Read the model definition and answer for the solid it produces. Units are mm, in the model's axes. A direction names the side the tool comes from. Round coordinates to 2 decimals unless told otherwise and drop trailing zeros. Loops run counter-clockwise (first coordinate to the right, second up) from the corner with the lowest first, then second, coordinate; pieces in that order, holes last. Notation, with made-up numbers: M -14.5,80 L 33.5,80 A20 cw 33.5,109 Z; hole C 2.25,8 d2. An arc over 180 degrees is marked long. Write each question's results on one line, items separated by ' | '.
from build123d import *

# Parameters (mm, degrees)
BOSS_EXTRUDE1_DEPTH          = 50.8
CUT_EXTRUDE1_START           = -50.8
CUT_EXTRUDE1_DEPTH           = 34.036
SKETCH10_W                   = 50.546
SKETCH10_H                   = 34.036
CUT_EXTRUDE3_DEPTH           = 20.734311378
CUT_EXTRUDE4_DEPTH           = 2.54
CUT_EXTRUDE5_DEPTH           = 7.874
FILLET1_R                    = 2.54
FILLET2_R                    = 2.54
CUT_EXTRUDE6_DEPTH           = 51.8
F_10_0_1935_DIAMETER_HOLE1_D = 4.9149
FILLET3_R                    = 2.54
CUT_EXTRUDE7_DEPTH           = 5.334
SKETCH18_W                   = 7.62
SKETCH18_H                   = 2.54


with BuildPart() as part:
    # Sketch1 → Boss-Extrude1 (new body)
    with BuildSketch(Plane(origin=(0, 0, 0), x_dir=(1, 0, 0), z_dir=(0, 1, 0))):
        with BuildLine():
            Line((63.017839503, -66.782093), (53.468205472, -26.506342671))
            Line((53.468205472, -26.506342671), (-35.875703335, -47.690346072))
            Line((-35.875703335, -47.690346072), (-26.326069304, -87.966096401))
            ThreePointArc((-26.326069304, -87.966096401), (21.184003401, -89.343908807), (63.017839503, -66.782093))
        make_face()
    extrude(amount=BOSS_EXTRUDE1_DEPTH)

    # Sketch2 → Cut-Extrude1 (cut)
    with BuildSketch(Plane(origin=(0, 50.8, 0), x_dir=(1, 0, 0), z_dir=(0, 1, 0)).offset(CUT_EXTRUDE1_START)):
        Polygon((19.413866358, -81.878324539), (49.046880649, -74.852150244), (42.542248899, -47.418750859), (-6.6401518, -59.08020778), (-0.13552005, -86.513607165), align=None)
    extrude(amount=CUT_EXTRUDE1_DEPTH, mode=Mode.SUBTRACT)

    # Sketch10 → Cut-Extrude3 (cut, through all)
    with BuildSketch(Plane(origin=(19.413866358, 0, 81.878324539), x_dir=(-0.973022607, 0, 0.230709788), z_dir=(-0.230709788, 0, -0.973022607))):
        with Locations((-5.1816, 17.018)):
            Rectangle(SKETCH10_W, SKETCH10_H)
    extrude(amount=-CUT_EXTRUDE3_DEPTH, mode=Mode.SUBTRACT)

    # Sketch11 → Cut-Extrude4 (cut)
    with BuildSketch(Plane.XZ.offset(-34.036)):
        Polygon((4.126655542, 64.024522649), (32.455610184, 56.972208264), (36.418920031, 72.892715879), (8.089965389, 79.945030264), align=None)
    extrude(amount=-CUT_EXTRUDE4_DEPTH, mode=Mode.SUBTRACT)

    # Sketch12 → Cut-Extrude5 (cut)
    with BuildSketch(Plane(origin=(0, 50.8, 0), x_dir=(1, 0, 0), z_dir=(0, 1, 0))):
        Polygon((-3.21042467, -90.775014105), (35.097475372, -81.69196977), (27.186436757, -48.327024572), (-11.121463285, -57.410068908), align=None)
    extrude(amount=-CUT_EXTRUDE5_DEPTH, mode=Mode.SUBTRACT)

    # Fillet1
    fillet1_edges = [part.edges().sort_by_distance(p)[0] for p in [
        (53.468205472, 25.4, 26.506342671),
    ]]
    fillet(fillet1_edges, radius=FILLET1_R)

    # Fillet2
    fillet2_edges = [part.edges().sort_by_distance(p)[0] for p in [
        (-35.875703335, 25.4, 47.690346072),
    ]]
    fillet(fillet2_edges, radius=FILLET2_R)

    # Sketch13 → Cut-Extrude6 (cut, through all)
    with BuildSketch(Plane(origin=(0, 50.8, 0), x_dir=(1, 0, 0), z_dir=(0, 1, 0))):
        Polygon((56.792853338, -82.364213599), (69.150240448, -79.434199297), (54.970742259, -19.631915037), (-50.56134592, -44.654237709), (-47.281500933, -58.487041918), (45.893200136, -36.394733549), align=None)
    extrude(amount=-CUT_EXTRUDE6_DEPTH, mode=Mode.SUBTRACT)

    # #10 (0.1935) Diameter Hole1 (through all)
    with Locations(Plane(origin=(0, 50.8, 0), x_dir=(1, 0, 0), z_dir=(0, 1, 0))):
        with Locations((-9.336173019, -54.694807642), (34.992334459, -45.467652744)):
            Hole(F_10_0_1935_DIAMETER_HOLE1_D / 2)

    # Fillet3
    fillet3_edges = [part.edges().sort_by_distance(p)[0] for p in [
        (-34.059094468, 25.4, 55.35192608),
        (45.893200136, 25.4, 36.394733549),
    ]]
    fillet(fillet3_edges, radius=FILLET3_R)

    # Sketch17 → Cut-Extrude7 (cut)
    with BuildSketch(Plane(origin=(0, 50.8, 0), x_dir=(1, 0, 0), z_dir=(0, 1, 0))):
        Polygon((-5.287837916, -82.013487021), (33.020062126, -72.930442686), (37.24926209, -90.767168294), (-1.058637951, -99.850212629), align=None)
    extrude(amount=-CUT_EXTRUDE7_DEPTH, mode=Mode.SUBTRACT)

    # Sketch18 → Cut-Revolve1 (revolve, cut)
    with BuildSketch(Plane(origin=(0, 0, 0), x_dir=(0, 1, 0), z_dir=(0.999925437, 0, -0.012211508))):
        with Locations((36.576, 90.551)):
            Rectangle(SKETCH18_W, SKETCH18_H)
    revolve(axis=Axis((0, 50.8, 0), (0, -1, 0)), mode=Mode.SUBTRACT)


solid = part.part
Item 1: The mould has two halves that part along X. Classify faces 1 (the face through (10, 50.8, 52)), 2 (the face through (50.553, 25.756, 56.048)), 3 (the face through (-9.016, 25.044, 52.258)): pulls with the +X half, pulls with the -X half, needs draft (parallel to the pull), parting line crosses it, or undercut.
Outcome:
face 1: needs draft | face 2: pulls with the +X half | face 3: undercut
Item 2: Straight lines are drawn through the part: line 1 (Y direction, x = -1, z = 64); line 2 (Y direction, x = 25.5, z = 73); line 3 (Z direction, x = 37, y = 48). For each, find the intervals that lie inside material, in ascending order.
Outcome:
line 1: y = 34.04 to 42.93 | line 2: y = 36.58 to 42.93 | line 3: z = 38.5 to 44.05, 46.88 to 84.04
Item 3: Flat-ended cylindrical pins translate along their axes: pin 1 (4 mm diameter, centred on y = 18, z = 74.5, fed in from -X); pin 2 (5 mm diameter, centred on x = 9.5, z = 88, fed in from +Y); pin 3 (1 mm diameter, centred on y = 43, z = 80.5, fed in from -X). Find the tip coordinate at first contact, or state that the pin passes through.
Outcome:
pin 1: stops at x = -29.99 | pin 2: stops at y = 45.47 | pin 3: stops at x = -28.21
Item 4: The part is cut by section C-C (z = 78.5). Determine the outline of the cut face in (x, y), plus the area to 3 significant figures.
Outcome:
outline: M -28.57,0 L -2.04,0 L -2.04,34.04 L 7.73,34.04 L 7.73,36.58 L 13.89,36.58 L 13.89,34.04 L 42.53,34.04 L 42.53,40.39 L 47.63,40.39 L 47.63,50.8 L 34.34,50.8 L 34.34,42.93 L -6.12,42.93 L -6.12,50.8 L -28.57,50.8 Z | area: 1,810 mm2
Item 5: The part is cut by section B-B (x = -15). Determine the outline of the cut face in (y, z), plus the area to 3 significant figures.
Outcome:
outline: M 0,50.83 L 50.8,50.83 L 50.8,90.59 L 40.39,90.59 L 40.39,88.01 L 32.77,88.01 L 32.77,90.59 L 0,90.59 Z | area: 2,000 mm2
Item 6: For faces 4 (the face through (15.86, 36.63, 87.86)), 5 (the face through (12, 42.926, 69)), 6 (the face through (52, 32.766, 74)), determine the directions among +Z, -Z, +X, -X, +Y, -Y from which every point of the face is accessible in a straight line to the end or side of a thin tool.
Outcome:
face 4: +Z | face 5: +Y | face 6: +Z, +X
Item 7: The part is cut by section D-D (y = 21). Determine the outline of the cut face in (x, z).
Outcome:
outline: M -33.47,57.82 A2.54 ccw -31.59,54.77 L 43.42,36.98 A2.54 ccw 46.48,38.87 L 54.74,73.72 A91.82 ccw 49.62,77.26 L 42.54,47.42 L -6.64,59.08 L 1.12,91.81 A91.82 ccw -26.33,87.97 Z; hole C -9.34,54.69 d4.91; hole C 34.99,45.47 d4.91
Item 8: The part is cut by section A-A (y = 42). Determine the outline of the cut face in (x, z), plus the area to 3 significant figures.
Outcome:
outline: M -33.47,57.82 A2.54 ccw -31.59,54.77 L 43.42,36.98 A2.54 ccw 46.48,38.87 L 54.74,73.72 A91.82 ccw -26.33,87.97 Z; hole C -9.34,54.69 d4.91; hole C 34.99,45.47 d4.91 | area: 3,450 mm2
